Geometry: see drawing. Coordinates: mm, zero at the bounding-box minimum. Round coordinates to 2 decimals unless told otherwise and drop trailing zeros. Loops run counter-clockwise (first coordinate to the right, second up) from the corner with the lowest first, then second, coordinate; pieces in that order, holes last. Notation, with made-up numbers: (15, 23.25) - (62, 23.25) arc R23 cw to (62, 49.25) - close; hole circle Ø7 at (9, 7). An arc over 180 degrees is marked (long way). Write item = value, one per line. Start each with the question number.
Item 1: Section D-D (y = 0.5). Return loops of the section in (x, z).
Item 2: Section A-A (x = 47). Return loops of the section in (y, z), plus the area to 3 significant figures.
Item 3: Line query: line 1 (Z direction, x = 51, y = 0.85); line 2 (Z direction, x = 49, y = 0.8); line 3 (X direction, y = 0.4, z = 98.25). Output: solid intervals per line, ascending. Write a range as from..to.
Item 4: Section C-C (z = 21.5). Return loops of the section in (x, y), plus the area to 3 significant figures.
Item 5: Section B-B (z = 51). Return loops of the section in (x, y), plus the area to 3 significant figures.
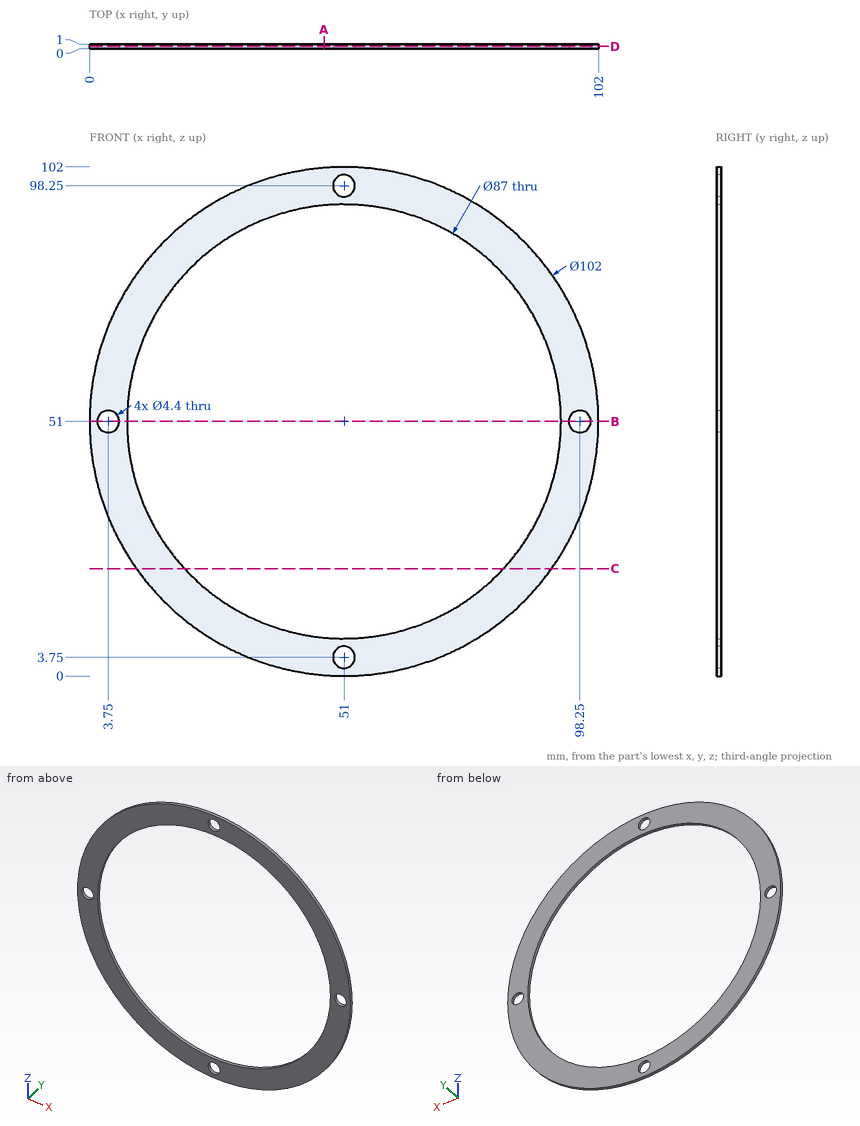
Taken from the geometry:
q1.outline = circle Ø102 at (51, 51); hole circle Ø4.4 at (3.75, 51); hole circle Ø87 at (51, 51); hole circle Ø4.4 at (51, 3.75); hole circle Ø4.4 at (51, 98.25); hole circle Ø4.4 at (98.25, 51)
q2.outline = (0, 0.16) - (1, 0.16) - (1, 7.68) - (0, 7.68) - close; (0, 94.32) - (1, 94.32) - (1, 101.84) - (0, 101.84) - close
q2.area = 15.1 mm^2
q3.line_1 = 0..1.55, 5.95..7.5, 94.5..96.05, 100.45..102
q3.line_2 = 0.04..2.83, 4.67..7.55, 94.45..97.33, 99.17..101.96
q3.line_3 = 31.81..48.8, 53.2..70.19
q4.outline = (9.4, 0) - (19.03, 0) - (19.03, 1) - (9.4, 1) - close; (82.97, 0) - (92.6, 0) - (92.6, 1) - (82.97, 1) - close
q4.area = 19.3 mm^2
q5.outline = (0, 0) - (1.55, 0) - (1.55, 1) - (0, 1) - close; (5.95, 0) - (7.5, 0) - (7.5, 1) - (5.95, 1) - close; (94.5, 0) - (96.05, 0) - (96.05, 1) - (94.5, 1) - close; (100.45, 0) - (102, 0) - (102, 1) - (100.45, 1) - close
q5.area = 6.20 mm^2
